Can you work these out from the model? Positions are in its coordinate system, mm. Face numbers are marked on the shaded views. A direction names the side the tool comes from. Coordinates: 2 decimals unless noted, no trailing zeros. Write each loop counter-clockwise with the first axis right and the second up, starting at its lowest first coordinate (ties: lowest second). Pieces come first, ordered by that corner, then holes. Notation, with made-up numbers: (-5, 59) - (15, 59) arc R28 ccw to (15, 79) - close; hole circle Ø4 at (30.5, -20.5). An arc over 180 degrees is marked (long way). Use one line per item in the form item = value. Start each with the question number.
(1) If we section it at D-D on x = -5.5: Please give me the cut outline in (y, z).
(2) If we section it at B-B on x = 13.08: Please give me the cut outline in (y, z), then the cut area to 3 significant figures.
(3) If we section it at A-A on y = 39: Please give me the cut outline in (x, z).
(4) If I drill on probe 1 along Y at (x, z) = (13.08, 2.8); probe 2 along X at (y, z) = (58, -1); probe 3 along Y at (x, z) = (13.08, -0.95), over which ranges is the centre line in solid material (lowest first)? Write a range as from..to.
(5) On a 3-axis mill with a long thin cutter (end or side, diameter ignored), from which of +Z, -Z, +X, -X, +Y, -Y can I reach the whole of each face in a straight line? I mean the marked faces 1, 2 and 3. Say none if no direction works.
(6) For pin 1 Ø11 at (x, y) = (13.08, 99.19) entering from +Z; pin 2 Ø2.5 at (y, z) = (19, -0.5) entering from -X; pin 3 Ø2 at (x, z) = (15, 2) entering from +Y, each with a flat end and sliding along its axis, tell me the tip position at first contact or that it passes through.
(7) If we section it at C-C on z = -2: Please give me the cut outline in (x, y), then the cut area to 3 significant figures.
```python
from build123d import *

# Parameters (mm, degrees)
ESTRUSIONE_ESTRUSIONE1_DEPTH                         = 4
TAGLIO_ESTRUSIONE1_DEPTH                             = 134.270896221
FORO_LAMATO_PER_BULLONE_M5_A_TESTA_ESAGO_D           = 5.5
FORO_LAMATO_PER_BULLONE_M5_A_TESTA_ESAGO_CBORE_D     = 12.238
FORO_LAMATO_PER_BULLONE_M5_A_TESTA_ESAGO_CBORE_DEPTH = 3.5


with BuildPart() as part:
    # Schizzo1 → Estrusione-Estrusione1 (new, symmetric)
    with BuildSketch(Plane.XY):
        with BuildLine():
            Line((0, 0), (0, 75))
            ThreePointArc((0, 75), (13.08, 126.690155022), (26.16, 75))
            Line((26.16, 75), (26.16, 0))
            Line((26.16, 0), (0, 0))
        make_face()
    extrude(amount=ESTRUSIONE_ESTRUSIONE1_DEPTH, both=True)

    # Schizzo2 → Taglio-Estrusione1 (cut, through all)
    with BuildSketch(Plane.XY.offset(4)):
        with BuildLine():
            Line((10.58, 12), (10.58, 80))
            ThreePointArc((10.58, 80), (13.08, 82.5), (15.58, 80))
            Line((15.58, 80), (15.58, 12))
            ThreePointArc((15.58, 12), (13.08, 9.5), (10.58, 12))
        make_face()
    extrude(amount=-TAGLIO_ESTRUSIONE1_DEPTH, mode=Mode.SUBTRACT)

    # Foro lamato per Bullone M5 a testa esagonale-1 (through all)
    with Locations(Plane.XY.offset(4)):
        with Locations((13.08, 99.190155022)):
            CounterBoreHole(FORO_LAMATO_PER_BULLONE_M5_A_TESTA_ESAGO_D / 2, FORO_LAMATO_PER_BULLONE_M5_A_TESTA_ESAGO_CBORE_D / 2, FORO_LAMATO_PER_BULLONE_M5_A_TESTA_ESAGO_CBORE_DEPTH)


solid = part.part
```
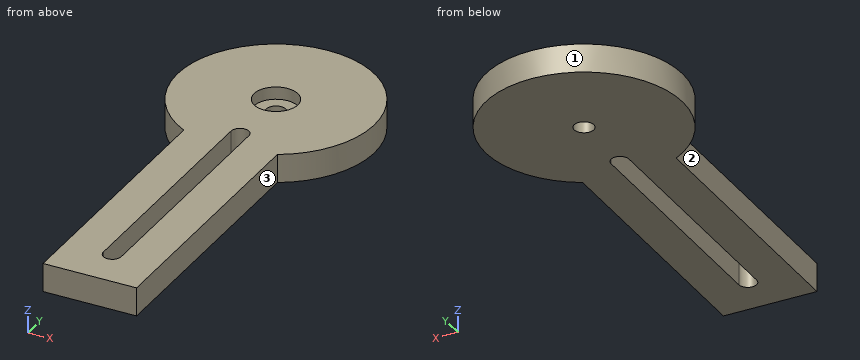
Reported:
q1.outline = (78.92, -4) - (119.46, -4) - (119.46, 4) - (78.92, 4) - close
q2.outline = (0, -4) - (9.5, -4) - (9.5, 4) - (0, 4) - close; (82.5, -4) - (96.44, -4) - (96.44, 0.5) - (93.07, 0.5) - (93.07, 4) - (82.5, 4) - close; (101.94, -4) - (126.69, -4) - (126.69, 4) - (105.31, 4) - (105.31, 0.5) - (101.94, 0.5) - close
q2.area = 362 mm2
q3.outline = (0, -4) - (10.58, -4) - (10.58, 4) - (0, 4) - close; (15.58, -4) - (26.16, -4) - (26.16, 4) - (15.58, 4) - close
q4.probe_1 = 0..9.5, 82.5..93.07, 105.31..126.69
q4.probe_2 = 0..10.58, 15.58..26.16
q4.probe_3 = 0..9.5, 82.5..96.44, 101.94..126.69
q5.face_1 = +Z, -Z
q5.face_2 = +Z, -Z, -X, -Y
q5.face_3 = +Z, -Z, +X, -Y
q6.pin_1 = 0.5
q6.pin_2 = 0
q6.pin_3 = 126.67
q7.outline = (0, 0) - (26.16, 0) - (26.16, 75) arc R27.5 ccw (long way) to (0, 75) - close; hole circle Ø5.5 at (13.08, 99.19); hole (10.58, 12) arc R2.5 ccw to (15.58, 12) - (15.58, 80) arc R2.5 ccw to (10.58, 80) - close
q7.area = 3,900 mm2
